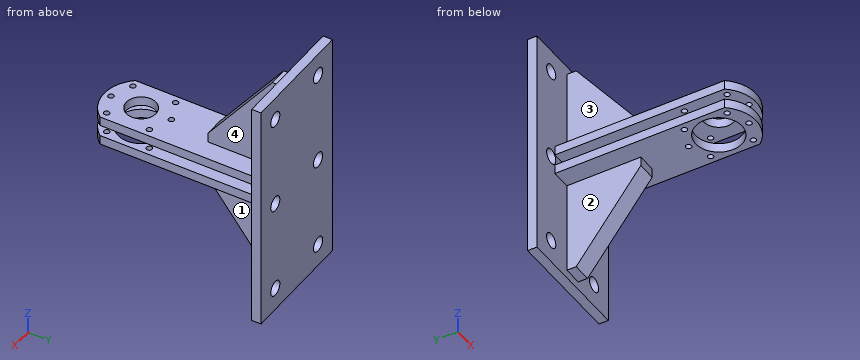
```python
from build123d import *

# Parameters (mm, degrees)
SKETCH1_R           = 3
SKETCH1_R_2         = 16
BOSS_EXTRUDE1_DEPTH = 10
SKETCH2_R           = 3.036946437
SKETCH2_R_2         = 3
SKETCH2_R_3         = 25
BOSS_EXTRUDE2_DEPTH = 10
SKETCH3_W           = 125
SKETCH3_H           = 250
BOSS_EXTRUDE3_DEPTH = 10
BOSS_EXTRUDE4_DEPTH = 10
SKETCH6_R           = 8
CUT_EXTRUDE1_DEPTH  = 10


with BuildPart() as part:
    # Sketch1 → Boss-Extrude1 (new body)
    with BuildSketch(Plane.XY):
        with BuildLine():
            Line((-31, -25.27844932), (-31, 157.52155068))
            Line((-31, 157.52155068), (31, 157.52155068))
            Line((31, 157.52155068), (31, -25.27844932))
            ThreePointArc((31, -25.27844932), (0, -40), (-31, -25.27844932))
        make_face()
        with Locations((0, 32.5)):
            Circle(SKETCH1_R, mode=Mode.SUBTRACT)
        with Locations((-22.980970389, 22.980970389)):
            Circle(SKETCH1_R, mode=Mode.SUBTRACT)
        with Locations((22.980970389, 22.980970389)):
            Circle(SKETCH1_R, mode=Mode.SUBTRACT)
        with Locations((22.980970389, -22.980970389)):
            Circle(SKETCH1_R, mode=Mode.SUBTRACT)
        with Locations((0, -32.5)):
            Circle(SKETCH1_R, mode=Mode.SUBTRACT)
        with Locations((-22.980970389, -22.980970389)):
            Circle(SKETCH1_R, mode=Mode.SUBTRACT)
        Circle(SKETCH1_R_2, mode=Mode.SUBTRACT)
    extrude(amount=BOSS_EXTRUDE1_DEPTH)



with BuildPart() as body_2:
    # Sketch2 → Boss-Extrude2 (new body)
    with BuildSketch(Plane(origin=(0, 0, -12), x_dir=(-1, 0, 0), z_dir=(0, 0, -1))):
        with BuildLine():
            Line((-31, 157.52155068), (31, 157.52155068))
            Line((31, 157.52155068), (31, -25.27844932))
            ThreePointArc((31, -25.27844932), (0, -40), (-31, -25.27844932))
            Line((-31, -25.27844932), (-31, 157.52155068))
        make_face()
        with Locations((0, 32.5)):
            Circle(SKETCH2_R, mode=Mode.SUBTRACT)
        with Locations((22.980970389, 22.980970389)):
            Circle(SKETCH2_R_2, mode=Mode.SUBTRACT)
        with Locations((-22.980970389, 22.980970389)):
            Circle(SKETCH2_R_2, mode=Mode.SUBTRACT)
        with Locations((22.980970389, -22.980970389)):
            Circle(SKETCH2_R_2, mode=Mode.SUBTRACT)
        with Locations((0, -32.5)):
            Circle(SKETCH2_R_2, mode=Mode.SUBTRACT)
        with Locations((-22.980970389, -22.980970389)):
            Circle(SKETCH2_R_2, mode=Mode.SUBTRACT)
        Circle(SKETCH2_R_3, mode=Mode.SUBTRACT)
    extrude(amount=BOSS_EXTRUDE2_DEPTH)


with BuildPart() as part_1:
    add(part.part)

    add(body_2.part)  # Boss-Extrude3 merges body 2
    # Sketch3 → Boss-Extrude3 (add)
    with BuildSketch(Plane(origin=(0, 157.52155068, 0), x_dir=(1, 0, 0), z_dir=(0, 1, 0))):
        with Locations((0, 6)):
            Rectangle(SKETCH3_W, SKETCH3_H)
    extrude(amount=BOSS_EXTRUDE3_DEPTH)

    # Sketch5 → Boss-Extrude4 (add, symmetric)
    with BuildSketch(Plane(origin=(0, 0, 0), x_dir=(0, 0, -1), z_dir=(1, 0, 0))):
        Polygon((22, 157.52155068), (122, 157.52155068), (122, 147.52155068), (32, 77.933321793), (22, 77.933321793), align=None)
        Polygon((-20, 77.933321793), (-10, 77.933321793), (-10, 157.52155068), (-110, 157.52155068), (-110, 147.52155068), align=None)
    extrude(amount=BOSS_EXTRUDE4_DEPTH, both=True)

    # Sketch6 → Cut-Extrude1 (cut)
    with BuildSketch(Plane(origin=(0, 167.52155068, 0), x_dir=(1, 0, 0), z_dir=(0, 1, 0))):
        with Locations((-37.5, 106)):
            Circle(SKETCH6_R)
        with Locations((37.5, 106)):
            Circle(SKETCH6_R)
        with Locations((37.5, 6)):
            Circle(SKETCH6_R)
        with Locations((37.5, -94)):
            Circle(SKETCH6_R)
        with Locations((-37.5, -94)):
            Circle(SKETCH6_R)
        with Locations((-37.5, 6)):
            Circle(SKETCH6_R)
    extrude(amount=-CUT_EXTRUDE1_DEPTH, mode=Mode.SUBTRACT)


solid = part_1.part
```
Design review of the part built by this model. Coordinates are the model's own, in mm. Face numbers are marked on the shaded views. A direction names the side the tool comes from. Give positions to 0.01 mm unless a question says otherwise; leave off trailing zeros. Loops run counter-clockwise (first coordinate to the right, second up) from the corner with the lowest first, then second, coordinate; pieces in that order, holes last. Notation, with made-up numbers: (-19, -13) -> (22, -13) arc R11 ccw to (22, 8) -> close; hole circle Ø1 at (24, 68). An arc over 180 degrees is marked (long way). One line per item, written item: value.
Q1. For pin 1 Ø8 at (x, y) = (3.5, 40.5) entering from -Z; pin 2 Ø3 at (x, z) = (3.5, 16.5) entering from -Y; pin 3 Ø3 at (x, y) = (2.5, 152.5) entering from -Z, all flat-tipped, find the tip position at first contact; note any pin that passes through.
Numbers:
pin 1: stops at z = -22
pin 2: stops at y = 77.93
pin 3: stops at z = -122
Q2. We need section C-C on z = -6. Give the boundary of the cut face in (x, y).
Numbers:
outline: (-62.5, 157.52) -> (-45.5, 157.52) -> (-45.5, 167.52) -> (-62.5, 167.52) -> close; (-29.5, 157.52) -> (29.5, 157.52) -> (29.5, 167.52) -> (-29.5, 167.52) -> close; (45.5, 157.52) -> (62.5, 157.52) -> (62.5, 167.52) -> (45.5, 167.52) -> close
Q3. We need section D-D on x = 6. Give the boundary of the cut face in (y, z).
Numbers:
outline: (-39.55, -22) -> (-24.27, -22) -> (-24.27, -12) -> (-39.55, -12) -> close; (-39.55, 0) -> (-14.83, 0) -> (-14.83, 10) -> (-39.55, 10) -> close; (14.83, 0) -> (157.52, 0) -> (157.52, -12) -> (24.27, -12) -> (24.27, -22) -> (77.93, -22) -> (77.93, -32) -> (147.52, -122) -> (157.52, -122) -> (157.52, -131) -> (167.52, -131) -> (167.52, 119) -> (157.52, 119) -> (157.52, 110) -> (147.52, 110) -> (77.93, 20) -> (77.93, 10) -> (14.83, 10) -> close
Q4. We need section B-B on x = -37.5. Give the boundary of the cut face in (y, z).
Numbers:
outline: (157.52, -131) -> (167.52, -131) -> (167.52, -114) -> (157.52, -114) -> close; (157.52, -98) -> (167.52, -98) -> (167.52, -14) -> (157.52, -14) -> close; (157.52, 2) -> (167.52, 2) -> (167.52, 86) -> (157.52, 86) -> close; (157.52, 102) -> (167.52, 102) -> (167.52, 119) -> (157.52, 119) -> close
Q5. We need section A-A on y = 32.5. Give the boundary of the cut face in (x, z).
Numbers:
outline: (-31, -22) -> (-3.04, -22) -> (-3.04, -12) -> (-31, -12) -> close; (-31, 0) -> (-3, 0) -> (-3, 10) -> (-31, 10) -> close; (3, 0) -> (31, 0) -> (31, 10) -> (3, 10) -> close; (3.04, -22) -> (31, -22) -> (31, -12) -> (3.04, -12) -> close
Q6. For L1, parallel to Z at x = -37, y = 163; L2, parallel to Y at x = 0, z = 6.25; L3, parallel to Z at x = 30, y = 47, list the stretches that pass through material, from the lowest coordinate up.
Numbers:
L1: z = -131 to -113.98, -98.02 to -13.98, 1.98 to 86.02, 101.98 to 119
L2: y = -40 to -35.5, -29.5 to -16, 16 to 29.5, 35.5 to 167.52
L3: z = -22 to -12, 0 to 10
Q7. Machinability: for the marked faces 1, 2, 3 and 4, which of the approach directions +Z, -Z, +X, -X, +Y, -Y give a long, thin tool a straight path to every point of the face, cutting with its end or side? Answer none if there is none.
Numbers:
face 1: -Z, +X, -Y
face 2: -Z, -X, -Y
face 3: +Z, -X, -Y
face 4: +Z, +X, -Y
